from build123d import *

# Parameters (mm, degrees)
SKETCH1_W           = 56.388
SKETCH1_H           = 45.72
BOSS_EXTRUDE1_DEPTH = 2.54
SKETCH2_W           = 2.7432
SKETCH2_H           = 19.05
BOSS_EXTRUDE2_DEPTH = 2.54
SKETCH3_W           = 19.05
SKETCH3_H           = 2.7432
CUT_EXTRUDE1_DEPTH  = 3.54


with BuildPart() as part:
    # Sketch1 → Boss-Extrude1 (new body)
    with BuildSketch(Plane(origin=(0, 0, 0), x_dir=(0, 0, -1), z_dir=(1, 0, 0))):
        Rectangle(SKETCH1_W, SKETCH1_H)
    extrude(amount=BOSS_EXTRUDE1_DEPTH)

    # Sketch2 → Boss-Extrude2 (add)
    with BuildSketch(Plane(origin=(2.54, 0, 0), x_dir=(0, 0, -1), z_dir=(1, 0, 0))):
        with Locations((-29.5656, 0)):
            Rectangle(SKETCH2_W, SKETCH2_H)
        with Locations((29.5656, 0)):
            Rectangle(SKETCH2_W, SKETCH2_H)
    extrude(amount=-BOSS_EXTRUDE2_DEPTH)

    # Sketch3 → Cut-Extrude1 (cut, through all)
    with BuildSketch(Plane(origin=(2.54, 0, 0), x_dir=(0, 0, -1), z_dir=(1, 0, 0))):
        with Locations((0, 21.4884)):
            Rectangle(SKETCH3_W, SKETCH3_H)
        with Locations((0, -14.7066)):
            Rectangle(SKETCH3_W, SKETCH3_H)
    extrude(amount=-CUT_EXTRUDE1_DEPTH, mode=Mode.SUBTRACT)


solid = part.part
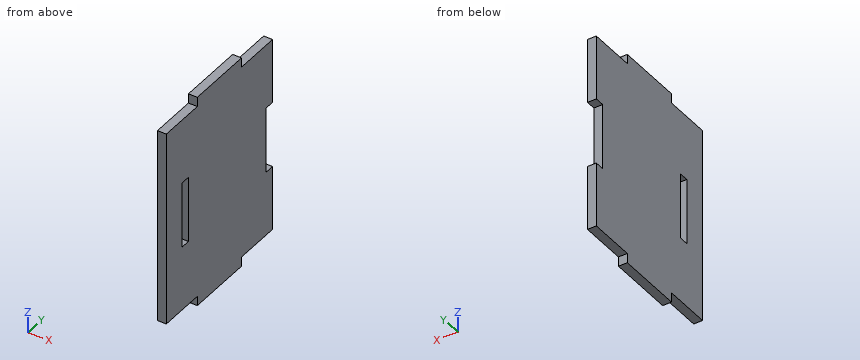
Here's how the part is built. I have some questions about the finished solid (model axes, mm). Round coordinates to 2 decimals unless told otherwise and drop trailing zeros. Order: outer loops, then holes, each group sorted by start corner. A loop starts at its lowest first (then second) coordinate and runs counter-clockwise, first axis right, second up. Notation, with made-up numbers: (47.5, 79.25) -> (52.5, 79.25) arc R27 ccw to (52.5, 111.25) -> close; hole circle Ø9 at (31.25, -2.5). An arc over 180 degrees is marked (long way). Use CSV: the item, a comma, the result in double quotes.
1. I want a section at B-B on x = 1.35. List the corners of the cut face in (y, z) for me (3 decimals).
Recorded:
outline,"(-22.86, -28.194) -> (-9.525, -28.194) -> (-9.525, -30.937) -> (9.525, -30.937) -> (9.525, -28.194) -> (22.86, -28.194) -> (22.86, -9.525) -> (20.117, -9.525) -> (20.117, 9.525) -> (22.86, 9.525) -> (22.86, 28.194) -> (9.525, 28.194) -> (9.525, 30.937) -> (-9.525, 30.937) -> (-9.525, 28.194) -> (-22.86, 28.194) -> close; hole (-16.078, -9.525) -> (-13.335, -9.525) -> (-13.335, 9.525) -> (-16.078, 9.525) -> close"
2. I'm going to push flat-ended pins straight in: P1, Ø10, axis at y = 13, z = 21, coming from the -X side; P2, Ø0.8, axis at x = 0.5, z = -29.5, coming from the +Y side (3 decimals); P3, Ø1.3, axis at x = 1, y = -14.5, coming from the +Z side; P4, Ø1.3, axis at x = 1, y = 15, coming from the -Z side. Where does each tip first touch, or does it pass through?
Recorded:
P1,"stops at x = 0"
P2,"stops at y = 9.525"
P3,"stops at z = 28.19"
P4,"stops at z = -28.19"
3. I need wall thicknesses on line 1 along Y through (x, z) = (2.2, -5) (3 decimals); line 2 along Z through (x, y) = (1.25, 20.5) (3 decimals); line 3 along Z through (x, y) = (2.2, -18). Which ranges of each line are inside material? Lowest first, please.
Recorded:
line 1,"y = -22.86 to -16.078, -13.335 to 20.117"
line 2,"z = -28.194 to -9.525, 9.525 to 28.194"
line 3,"z = -28.19 to 28.19"
4. I want a section at A-A on z = -3. List the corners of the cut face in (x, y) for me (3 decimals).
Recorded:
outline,"(0, -22.86) -> (2.54, -22.86) -> (2.54, -16.078) -> (0, -16.078) -> close; (0, -13.335) -> (2.54, -13.335) -> (2.54, 20.117) -> (0, 20.117) -> close"
5. I want a section at C-C on y = 10.5. List the corners of the cut face in (x, z) for me.
Recorded:
outline,"(0, -28.19) -> (2.54, -28.19) -> (2.54, 28.19) -> (0, 28.19) -> close"
